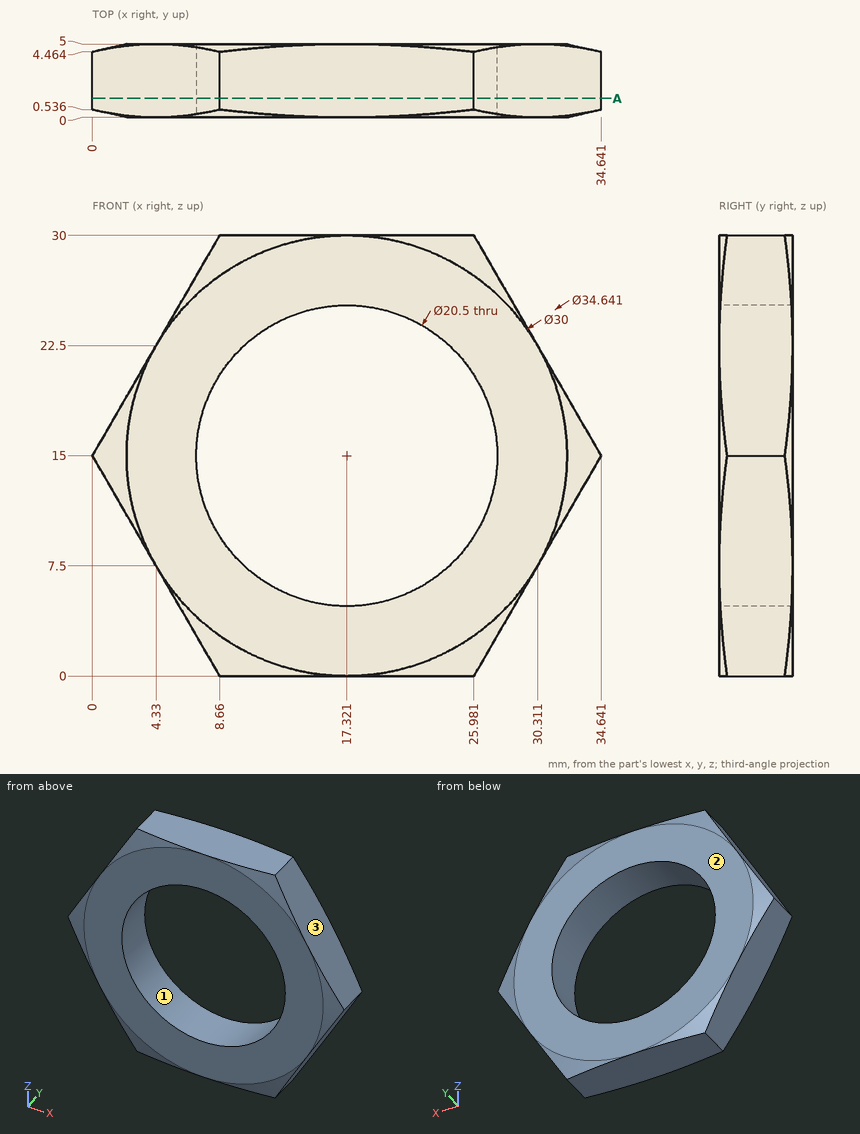
Part print with two shaded views. Sizes in mm from the minimum x, y, z corner. Give positions to 0.01 mm unless a question says otherwise; leave off trailing zeros. Loops run counter-clockwise (first coordinate to the right, second up) from the corner with the lowest first, then second, coordinate; pieces in that order, holes last. Notation, with made-up numbers: (24, -11) - (82, -11) arc R31 cw to (82, 17) - close; hole circle Ø6 at (27, 20). An arc over 180 degrees is marked (long way). Put each result on its own line as item: value.
Q1. Slice it at A-A (y = 1.3). Give the cut face in (x, z).
Filled in:
outline: (0, 15) - (8.66, 0) - (25.98, 0) - (34.64, 15) - (25.98, 30) - (8.66, 30) - close; hole circle Ø20.5 at (17.32, 15)
Q2. Probe line 1 along X through (y, z) = (2.05, 15); line 2 along X through (y, z) = (1.55, 8.75) (1 decimal); line 3 along Z through (x, y) = (18, 3.05). List the from-to ranges inside material, lowest first.
Filled in:
line 1: x = 0 to 7.07, 27.57 to 34.64
line 2: x = 3.6 to 9.2, 25.4 to 31
line 3: z = 0 to 4.77, 25.23 to 30
Q3. Mould opens along X. For the marked faces 1, 2 and 3 say: pulls with the +X half, pulls with the -X half, needs draft (parallel to the pull), parting line crosses it, or undercut.
Filled in:
face 1: undercut
face 2: needs draft
face 3: pulls with the +X half
Q4. Flat gauge pins, fed straight in: pin 1 (1 mm diameter, centred on x = 10, z = 3, fed in from -Y); pin 2 (3 mm diameter, centred on y = 2.5, z = 9.5, fed in from +X). Where does each tip first touch, or does it go through?
Filled in:
pin 1: stops at y = 0
pin 2: stops at x = 32.33
